Geometry: final body of the model. Coordinates: model frame, mm. A direction names the side the tool comes from. Coordinates: 2 decimals unless noted, no trailing zeros. Order: outer loops, then holes, each group sorted by start corner. A loop starts at its lowest first (then second) coordinate and runs counter-clockwise, first axis right, second up. Notation, with made-up numbers: M 22.5,46 L 62.5,46 A14 ccw 62.5,51 Z; hole C -13.5,81 d5. An arc over 180 degrees is marked long. Write item = value, one per line.
Autodesk Inventor part; units mm, degrees
ref_plane "YZ Plane" through (0, 0, 0) normal (1, 0, 0) x (0, 1, 0)
ref_plane "XZ Plane" through (0, 0, 0) normal (0, 1, 0) x (-1, 0, 0)
ref_plane "XY Plane" through (0, 0, 0) normal (0, 0, 1) x (1, 0, 0)
sketch "Szkic1" plane through (0, 0, 0) normal (0, 1, 0) x (-1, 0, 0)
  line L0 (0, 0) -> (3, 0)
  line L1 (3, 0) -> (3, -22)
  line L2 (3, -22) -> (0, -22)
  line L3 (0, -22) -> (0, 0)
  line L4 (0, 0) -> (-3, 0)
  line L5 (-3, 0) -> (-3, -5)
  line L6 (-3, -5) -> (0, -5)
  line L7 (0, -5) -> (0, 0)
  line L8 (0, -22) -> (-20, -22)
  line L9 (-20, -22) -> (-20, -19)
  line L10 (-20, -19) -> (0, -19)
  line L11 (0, -19) -> (0, -22)
  dimension "d0" = 3
  dimension "d1" = 22
  dimension "d2" = 3
  dimension "d3" = 5
  dimension "d4" = 20
  dimension "d5" = 3
extrude "Wyciągnięcie proste1" add sketch "Szkic1" along normal blind 8
sketch "Szkic2" plane through (0, 0, -19) normal (0, 0, 1) x (1, 0, 0)
  line L0 (20, 0) -> (20, 8)
  line L1 (20, 0) -> (0, 8)
  line L2 (20, 8) -> (-3, 8)
  point P0 (0, 0)
extrude "Wyciągnięcie proste2" cut sketch "Szkic2" against normal blind 3
sketch "Szkic3" plane through (-3, 0, 0) normal (0, 0, 1) x (1, 0, 0)
  line L0 (0, 0) -> (0, 8)
  line L1 (0, 0) -> (6, 0)
  line L2 (6, 0) -> (6, 8)
  line L3 (6, 8) -> (0, 8)
  line L4 (0, 8) -> (0, 0)
  point P0 (3, 0)
extrude "Wyciągnięcie proste3" add sketch "Szkic3" along normal blind 4.2
sketch "Szkic4" plane through (3, 0, -5) normal (0, 0, -1) x (-1, 0, 0)
  line L0 (0, 0) -> (0, 8)
  line L1 (3, 0) -> (3, 8)
  line L2 (0, 8) -> (3, 8)
  line L3 (3, 8) -> (3, 0)
  line L4 (3, 0) -> (0, 0)
  line L5 (0, 0) -> (0, 8)
extrude "Wyciągnięcie proste4" cut sketch "Szkic4" against normal blind 3.2
sketch "Szkic6" plane through (3, 0, 4.2) normal (1, 0, 0) x (0, 0, -1)
  line L0 (0, 8) -> (0, 0)
  line L1 (23.2, 0) -> (6, 0)
  line L2 (0, 8) -> (6, 8)
  line L3 (6, 8) -> (6, 0)
  line L4 (6, 0) -> (0, 0)
  line L5 (0, 0) -> (0, 8)
  point P0 (4.2, 0)
extrude "Wyciągnięcie proste7" add sketch "Szkic6" along normal blind 2
sketch "Szkic7" plane through (0, 8, 0) normal (0, 1, 0) x (1, 0, 0)
  circle A0 centre (1, -1.2) radius 2
  line L0 (5, 1.8) -> (5, -4.2)
  line L1 (-3, -4.2) -> (5, -4.2)
  line L2 (-3, 22) -> (-3, -4.2)
  line L3 (5, -4.2) -> (-3, -4.2)
  line L4 (-3, -4.2) -> (-3, 1.8)
  line L5 (-3, 1.8) -> (5, 1.8)
  line L6 (5, 1.8) -> (5, -4.2)
  point P0 (0, 0)
  dimension "d23" = 4
  dimension "d24" = 4
  dimension "d25" = 3
extrude "Wyciągnięcie proste8" cut sketch "Szkic7" against normal blind 8 contours A0
extrude "Wyciągnięcie proste9" cut sketch "Szkic7" against normal blind 5 contours A0 | L0 L1 L2 L5
sketch "Szkic8" plane through (5, 0, 4.2) normal (1, 0, 0) x (0, 0, -1)
  line L0 (0, 3) -> (0, 0)
  line L1 (23.2, 0) -> (6, 0)
  line L2 (0, 3) -> (6, 3)
  line L3 (6, 3) -> (6, 0)
  line L4 (6, 0) -> (0, 0)
  line L5 (0, 0) -> (0, 3)
  point P0 (4.2, 0)
extrude "Wyciągnięcie proste10" cut sketch "Szkic8" against normal blind 1
sketch "Szkic9" plane through (-3, 0, -22) normal (0, 0, -1) x (-1, 0, 0)
  line L0 (-3, 8) -> (-23, 0)
  line L1 (-23, 0) -> (-23, 3.137)
  line L2 (-3, 8) -> (-13, 8)
  line L3 (-13, 8) -> (-23, 3.137)
  point P0 (-3, 0)
  dimension "d32" = 3.137
extrude "Wyciągnięcie proste11" add sketch "Szkic9" against normal blind 3
sketch "Szkic10" plane through (0, 0, -19) normal (1, 0, 0) x (0, 0, -1)
  line L0 (0, 0) -> (-17.2, 0)
  line L1 (-17.2, 0) -> (-4.28, 0)
  line L2 (-4.28, 0) -> (-4.28, 1.5)
  line L3 (-4.28, 1.5) -> (-17.2, 1.5)
  line L4 (-17.2, 1.5) -> (-17.2, 0)
  point P0 (-19, 0)
  point P1 (-4.28, 0)
  dimension "d35" = 12.92
  dimension "d36" = 1.5
extrude "Wyciągnięcie proste12" add sketch "Szkic10" along normal blind 8.26
sketch "Szkic11" plane through (0, 1.5, -1.8) normal (0, 1, 0) x (1, 0, 0)
  circle A0 centre (4.8, 10.17) radius 1.55
  line L0 (4, 0) -> (8.26, 0)
  line L1 (0, 0) -> (0, 17.2)
  point P0 (0, -1.8)
  dimension "d39" = 3.1
  dimension "d40" = 10.17
  dimension "d41" = 4.8
extrude "Wyciągnięcie proste13" cut sketch "Szkic11" against normal blind 2
fillet "Fillet1" radius 3 1 edges at (4, 1.5, 4.2)
sketch "Szkic12" plane through (0, 1.5, -1.8) normal (0, 1, 0) x (1, 0, 0)
  circle A0 centre (4.8, 10.17) radius 1.55
  line L0 (0, 0) -> (0, 12.92)
  line L1 (4, 0) -> (0, 0)
  line L2 (4, 0) -> (8.26, 0)
  line L3 (8.26, 12.92) -> (8.26, 0)
  line L4 (0, 12.92) -> (8.26, 12.92)
  point P0 (0, -1.8)
extrude "Wyciągnięcie proste14" add sketch "Szkic12" along normal blind 1
sketch "Szkic13" plane through (0, 0, 0) normal (0, -1, 0) x (1, 0, 0)
  line L0 (8.26, -1.8) -> (8.26, -14.72)
  line L1 (8.26, -14.72) -> (0, -14.72)
  line L2 (0, -1.8) -> (0, -14.72)
  line L3 (4, -1.8) -> (0, -1.8)
  line L4 (4, -1.8) -> (8.26, -1.8)
  circle A0 centre (4.8, -11.97) radius 1.55
  point P0 (0, 0)
extrude "Wyciągnięcie proste15" cut sketch "Szkic13" against normal blind 1
properties part number "rfmw" material "Tworzywo sztuczne PET"
1) Section D-D, the plane z = 2. Return loops of the section in (x, y).
Numbers:
outline = M -3,0 L -0.83,0 L -0.83,3 L -3,3 Z; M 2.83,0 L 3.89,0 L 3.89,3 L 2.83,3 Z
2) Mould query, pull axis Z, two halves, no side actions, for faces 6 (the face through (-0.4, 8, -14.2)), 7 (the face through (4, 1, -8)), 8 (the face through (6, 2, -1.8)). Classes: pulls with the +Z half, pulls with the -Z half, needs draft (parallel to the pull), parting line crosses it, or undercut.
Numbers:
face_6 = needs draft
face_7 = undercut
face_8 = pulls with the +Z half
3) Section B-B, the plane x = 4.8. Return loops of the section in (y, z).
Numbers:
outline = M 0,-22 L 8,-22 L 8,-19 L 0,-19 Z; M 1,-14.72 L 2.5,-14.72 L 2.5,-13.52 L 1,-13.52 Z; M 1,-10.42 L 2.5,-10.42 L 2.5,-1.8 L 1,-1.8 Z
4) Set-up query: faces 1 (the face through (4, 2, 0)), 2 (the face through (8, 4, -19)), 3 (the face through (4, 2.5, -8)), 4 (the face through (-2, 6, -1.8)), 5 (the face through (2, 0.5, -1.8)). Return all of +Z, -Z, +X, -X, +Y, -Y with unobstructed straight access to the full face (end or side cutting, diameter ignored); none if empty.
Numbers:
face_1 = +Z, +X, +Y, -Y
face_2 = +X, +Y, -Y
face_3 = +X, +Y
face_4 = +Z, +X, -X, +Y
face_5 = +X, -Y
5) Pin query (flat end, axial travel): pin 1 (6.5 mm diameter, centred on x = 5, z = -10, fed in from +Y); pin 2 (1.6 mm diameter, centred on y = 2, z = -6, fed in from +X); pin 3 (3 mm diameter, centred on x = 4.8, z = -11.97, fed in from -Y); pin 4 (0.9 mm diameter, centred on x = -1, y = 4.5, fed in from +Z). Return the tip coordinate at first contact, or that it passes through.
Numbers:
pin_1 = 2.5
pin_2 = 8.26
pin_3 = through
pin_4 = -1.8
6) Line query: L1, parallel to Z at x = 1, y = 1.7; L2, parallel to X at y = 1.1, z = 1.2; L3, parallel to Z at x = 1, y = 0.75. Output: solid intervals per line, ascending.
Numbers:
L1 = -22 to -19, -14.72 to -0.8, 3.2 to 4.2
L2 = -3 to -1, 3 to 4
L3 = -22 to -19, -1.8 to -0.8, 3.2 to 4.2
7) Section A-A, the plane z = -11.97. Return loops of the section in (x, y), and give its area (3 significant figures).
Numbers:
outline = M -3,0 L 0,0 L 0,1 L 3.25,1 L 3.25,2.5 L 0,2.5 L 0,8 L -3,8 Z; M 6.35,1 L 8.26,1 L 8.26,2.5 L 6.35,2.5 Z
area = 31.7 mm²
8) Section C-C, the plane z = -8.5. Return loops of the section in (x, y), and give its area (3 significant figures).
Numbers:
outline = M -3,0 L 0,0 L 0,1 L 8.26,1 L 8.26,2.5 L 0,2.5 L 0,8 L -3,8 Z
area = 36.4 mm²
